Autodesk Fusion 360 part; units mm, degrees
sketch "Sketch1" plane through (0, 0, 0) normal (0, 0, 1) x (1, 0, 0)
  circle A0 centre (0, 0) radius 0.75
  dimension "d1" = 1.5
extrude "Extrude1" add sketch "Sketch1" along normal blind 33
sketch "Sketch2" plane through (0, 0, 33) normal (0, 0, 1) x (-1, 0, 0)
  circle A0 centre (0, 0) radius 0.75
  circle A1 centre (0, 0) radius 1.5
  dimension "d4" = 3
extrude "Extrude2" add sketch "Sketch2" against normal blind 1.5
fillet "Fillet1" radius 0.5 1 edges at (1.3985, 0.5424, 33)
fillet "Fillet2" radius 0.2 1 edges at (1.3985, -0.5424, 31.5)
sketch "Sketch3" plane through (0, 0, 33) normal (0, 0, 1) x (-1, 0, 0)
  circle A0 centre (0, 0) radius 1
  line L0 (0.6, 0.15) -> (-0.6, 0.15)
  arc A1 (-0.6, 0.15) -> (-0.6, -0.15) centre (-0.6, 0) ccw
  line L1 (-0.6, -0.15) -> (0.6, -0.15)
  arc A2 (0.6, -0.15) -> (0.6, 0.15) centre (0.6, 0) ccw
  line L2 (0.6, 0) -> (-0.6, 0) construction
  line L3 (-0.15, 0.6) -> (-0.15, -0.6)
  arc A3 (-0.15, -0.6) -> (0.15, -0.6) centre (0, -0.6) ccw
  line L4 (0.15, -0.6) -> (0.15, 0.6)
  arc A4 (0.15, 0.6) -> (-0.15, 0.6) centre (0, 0.6) ccw
  line L5 (0, 0.6) -> (0, -0.6) construction
  dimension "d11" = 0.3
  dimension "d12" = 1.2
  dimension "d13" = 0.3
  dimension "d14" = 1.2
extrude "Extrude3" cut sketch "Sketch3" against normal blind 1.2 contours L0 L1 A2 L4 | L0 L1 L3 L4 | L0 L3 L4 A4 | L0 A1 L1 L3 | L1 L3 A3 L4
fillet "Fillet3" radius 0.3 1 edges at (-0.6992, -0.2712, 0)
Work out the finished part from the listing and answer in its coordinate system (mm). Round coordinates to 2 decimals unless told otherwise and drop trailing zeros. Write each loop counter-clockwise with the first axis right and the second up, starting at its lowest first coordinate (ties: lowest second). Pieces come first, ordered by that corner, then holes.
1) Consider probe 1 along Y at (x, z) = (0, 4.5); probe 2 along X at (y, z) = (0.1, 29); probe 3 along Z at (x, y) = (0.5, 0.8). Determine where each line is inside the solid, lowest interval first.
2) A cutting plane is placed at A-A on z = 18.5. Determine the outline of the cut face in (x, y).
3) Flat-ended cylindrical pins translate along their axes: P1, Ø0.5, axis at y = -0.5, z = 32.5, coming from the +X side; P2, Ø0.5, axis at x = 0.5, z = 32.5, coming from the +Y side. Find the tip coordinate at first contact, or state that the pin passes through.
4) Determine the mould class of faces 1 (the face through (0, 0, 31.8)), 2 (the face through (0, 0, 0)), 3 (the face through (1.5, -0.07, 32.11)) for opening direction Y: pulls with the +Y half, pulls with the -Y half, needs draft (parallel to the pull), parting line crosses it, or undercut.
Entries:
1. probe 1: y = -0.75 to 0.75
1. probe 2: x = -0.74 to 0.74
1. probe 3: z = 31.5 to 33
2. outline: circle Ø1.5 at (0, 0)
3. P1: stops at x = 1.48
3. P2: stops at y = 1.48
4. face 1: undercut
4. face 2: needs draft
4. face 3: parting line crosses it
